```python
from build123d import *

# Parameters (mm, degrees)
SKETCH5_R           = 2.1
BOSS_EXTRUDE1_DEPTH = 125


with BuildPart() as part:
    # Sketch5 → Boss-Extrude1 (new body, symmetric)
    with BuildSketch(Plane(origin=(0, 0, 0), x_dir=(0, 0, -1), z_dir=(1, 0, 0))):
        with BuildLine():
            Line((-19.998019485, 4.9), (-18.198019485, 3.1))
            Line((-18.198019485, 3.1), (-18.198019485, 5.499339828))
            Line((-18.198019485, 5.499339828), (-16.558019485, 5.499339828))
            Line((-16.558019485, 5.499339828), (-13.9, 2.841320344))
            Line((-13.9, 2.841320344), (-13.9, -2.838679656))
            Line((-13.9, -2.838679656), (-16.558019485, -5.496699141))
            Line((-16.558019485, -5.496699141), (-18.198019485, -5.496699141))
            Line((-18.198019485, -5.496699141), (-18.198019485, -3.1))
            Line((-18.198019485, -3.1), (-19.998019485, -4.9))
            Line((-19.998019485, -4.9), (-19.998019485, -9))
            ThreePointArc((-19.998019485, -9), (-19.705126266, -9.707106781), (-18.998019485, -10))
            Line((-18.998019485, -10), (-14.9, -10))
            Line((-14.9, -10), (-13.1, -8.2))
            Line((-13.1, -8.2), (-15.5, -8.2))
            Line((-15.5, -8.2), (-15.5, -6.56))
            Line((-15.5, -6.56), (-12.84, -3.9))
            Line((-12.84, -3.9), (-7.16, -3.9))
            Line((-7.16, -3.9), (-4.5, -6.56))
            Line((-4.5, -6.56), (-4.5, -8.2))
            Line((-4.5, -8.2), (-6.9, -8.2))
            Line((-6.9, -8.2), (-5.1, -10))
            Line((-5.1, -10), (5.1, -10))
            Line((5.1, -10), (6.9, -8.2))
            Line((6.9, -8.2), (4.496038969, -8.2))
            Line((4.496038969, -8.2), (4.496038969, -6.56))
            Line((4.496038969, -6.56), (7.156038969, -3.9))
            Line((7.156038969, -3.9), (12.836038969, -3.9))
            Line((12.836038969, -3.9), (15.496038969, -6.56))
            Line((15.496038969, -6.56), (15.496038969, -8.2))
            Line((15.496038969, -8.2), (13.1, -8.2))
            Line((13.1, -8.2), (14.9, -10))
            Line((14.9, -10), (19.001980515, -10))
            ThreePointArc((19.001980515, -10), (19.709087297, -9.707106781), (20.001980515, -9))
            Line((20.001980515, -9), (20.001980515, -4.9))
            Line((20.001980515, -4.9), (18.201980515, -3.1))
            Line((18.201980515, -3.1), (18.201980515, -5.504621202))
            Line((18.201980515, -5.504621202), (16.561980515, -5.504621202))
            Line((16.561980515, -5.504621202), (13.9, -2.842640687))
            Line((13.9, -2.842640687), (13.9, 2.837359313))
            Line((13.9, 2.837359313), (16.561980515, 5.499339828))
            Line((16.561980515, 5.499339828), (18.201980515, 5.499339828))
            Line((18.201980515, 5.499339828), (18.201980515, 3.1))
            Line((18.201980515, 3.1), (20.001980515, 4.9))
            Line((20.001980515, 4.9), (20.001980515, 9))
            ThreePointArc((20.001980515, 9), (19.709087297, 9.707106781), (19.001980515, 10))
            Line((19.001980515, 10), (14.9, 10))
            Line((14.9, 10), (13.1, 8.2))
            Line((13.1, 8.2), (15.501320344, 8.2))
            Line((15.501320344, 8.2), (15.501320344, 6.56))
            Line((15.501320344, 6.56), (12.841320344, 3.9))
            Line((12.841320344, 3.9), (7.161320344, 3.9))
            Line((7.161320344, 3.9), (4.501320344, 6.56))
            Line((4.501320344, 6.56), (4.501320344, 8.2))
            Line((4.501320344, 8.2), (6.9, 8.2))
            Line((6.9, 8.2), (5.1, 10))
            Line((5.1, 10), (-5.1, 10))
            Line((-5.1, 10), (-6.9, 8.2))
            Line((-6.9, 8.2), (-4.501320344, 8.2))
            Line((-4.501320344, 8.2), (-4.501320344, 6.56))
            Line((-4.501320344, 6.56), (-7.161320344, 3.9))
            Line((-7.161320344, 3.9), (-12.841320344, 3.9))
            Line((-12.841320344, 3.9), (-15.501320344, 6.56))
            Line((-15.501320344, 6.56), (-15.501320344, 8.2))
            Line((-15.501320344, 8.2), (-13.1, 8.2))
            Line((-13.1, 8.2), (-14.9, 10))
            Line((-14.9, 10), (-18.998019485, 10))
            ThreePointArc((-18.998019485, 10), (-19.705126266, 9.707106781), (-19.998019485, 9))
            Line((-19.998019485, 9), (-19.998019485, 4.9))
        make_face()
        with Locations((-10, 0)):
            Circle(SKETCH5_R, mode=Mode.SUBTRACT)
        with Locations((10, 0)):
            Circle(SKETCH5_R, mode=Mode.SUBTRACT)
        Polygon((6.1, -2.84), (6.1, 2.84), (2.7, 6.24), (2.7, 8.2), (-2.7, 8.2), (-2.7, 6.24), (-6.1, 2.84), (-6.1, -2.84), (-2.7, -6.24), (-2.7, -8.2), (2.7, -8.2), (2.7, -6.24), align=None, mode=Mode.SUBTRACT)
        with BuildLine():
            Line((16.571320344, 8.2), (18.001980515, 8.2))
            ThreePointArc((18.001980515, 8.2), (18.143401872, 8.141421356), (18.201980515, 8))
            Line((18.201980515, 8), (18.201980515, 6.569339828))
            ThreePointArc((18.201980515, 6.569339828), (18.078517202, 6.384563922), (17.860559159, 6.427918472))
            Line((17.860559159, 6.427918472), (16.429898987, 7.858578644))
            ThreePointArc((16.429898987, 7.858578644), (16.386544437, 8.076536686), (16.571320344, 8.2))
        make_face(mode=Mode.SUBTRACT)
        with BuildLine():
            Line((16.571320344, -8.2), (18.001980515, -8.2))
            ThreePointArc((18.001980515, -8.2), (18.143401872, -8.141421356), (18.201980515, -8))
            Line((18.201980515, -8), (18.201980515, -6.569339828))
            ThreePointArc((18.201980515, -6.569339828), (18.078517202, -6.384563922), (17.860559159, -6.427918472))
            Line((17.860559159, -6.427918472), (16.429898987, -7.858578644))
            ThreePointArc((16.429898987, -7.858578644), (16.386544437, -8.076536686), (16.571320344, -8.2))
        make_face(mode=Mode.SUBTRACT)
        with BuildLine():
            Line((-17.860559159, 6.427918472), (-16.429898987, 7.858578644))
            ThreePointArc((-16.429898987, 7.858578644), (-16.386544437, 8.076536686), (-16.571320344, 8.2))
            Line((-16.571320344, 8.2), (-18.001980515, 8.2))
            ThreePointArc((-18.001980515, 8.2), (-18.143401872, 8.141421356), (-18.201980515, 8))
            Line((-18.201980515, 8), (-18.201980515, 6.569339828))
            ThreePointArc((-18.201980515, 6.569339828), (-18.078517202, 6.384563922), (-17.860559159, 6.427918472))
        make_face(mode=Mode.SUBTRACT)
        with BuildLine():
            Line((-16.571320344, -8.2), (-18.001980515, -8.2))
            ThreePointArc((-18.001980515, -8.2), (-18.143401872, -8.141421356), (-18.201980515, -8))
            Line((-18.201980515, -8), (-18.201980515, -6.569339828))
            ThreePointArc((-18.201980515, -6.569339828), (-18.078517202, -6.384563922), (-17.860559159, -6.427918472))
            Line((-17.860559159, -6.427918472), (-16.429898987, -7.858578644))
            ThreePointArc((-16.429898987, -7.858578644), (-16.386544437, -8.076536686), (-16.571320344, -8.2))
        make_face(mode=Mode.SUBTRACT)
    extrude(amount=BOSS_EXTRUDE1_DEPTH, both=True)


solid = part.part
```
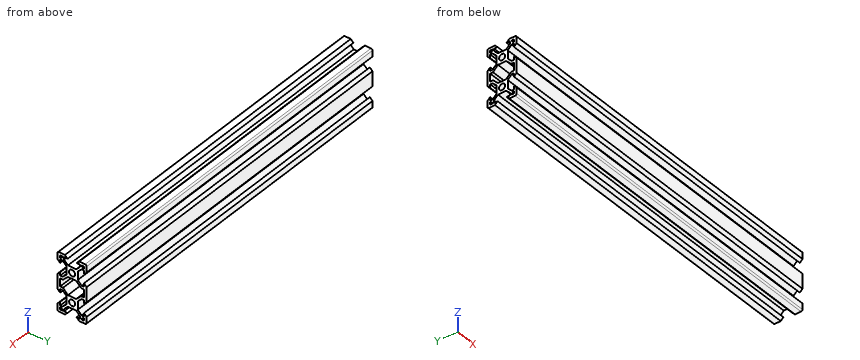
Geometry check sheet. Reference: the model listing, model coordinates, mm. Coordinates: 2 decimals unless noted, no trailing zeros. Order: outer loops, then holes, each group sorted by start corner. A loop starts at its lowest first (then second) coordinate and runs counter-clockwise, first axis right, second up. Notation, with made-up numbers: M -23.5,34 L 3.5,34 A16 ccw 3.5,60 Z; hole C -17.75,73.5 d5. An arc over 180 degrees is marked long. One line per question, with ' | ' between items. Start each with the question number.
Item 1: Material ranges on L1, parallel to Y at x = 16, z = -16; L2, parallel to Y at x = 55.5, z = -10; L3, parallel to Z at x = -43.5, y = -8.5, recorded low to high. Write a range as [from, to].
Item 2: Cross-section at A-A on y = 0. Enter the section's corners in (x, z), then the cut area to 3 significant figures.
Item 3: Gauge pin test, flat ends, axial feed: pin 1 (1.2 mm diameter, centred on x = -34.5, y = -4, fed in from +Z); pin 2 (2 mm diameter, centred on x = 70.5, z = -11, fed in from +Y); pin 3 (1 mm diameter, centred on x = 71.5, z = 11, fed in from -Y). Record the tip position at first contact, or that the pin passes through.
Item 4: Cross-section at C-C on x = -38.5. State how many separate pieces and enclosed holes the cut face has, then the cut area to 3 significant figures.
Item 5: Cross-section at B-B on z = 10. Enter the section's corners in (x, y), then the cut area to 3 significant figures.
Findings:
1) L1: y = [-10, -4.94], [4.94, 10] | L2: y = [-3.9, -2.1], [2.1, 3.9] | L3: z = [-20, -13.4], [-6.6, 6.6], [13.4, 20]
2) outline: M -125,-13.9 L 125,-13.9 L 125,-12.1 L -125,-12.1 Z; M -125,-7.9 L 125,-7.9 L 125,-6.1 L -125,-6.1 Z; M -125,6.1 L 125,6.1 L 125,7.9 L -125,7.9 Z; M -125,12.1 L 125,12.1 L 125,13.9 L -125,13.9 Z | area: 1,800 mm²
3) pin 1: stops at z = 19.7 | pin 2: stops at y = 3.9 | pin 3: stops at y = -3.9
4) separate pieces: 1 | enclosed holes: 7 | area: 285 mm²
5) outline: M -125,-3.9 L 125,-3.9 L 125,-2.1 L -125,-2.1 Z; M -125,2.1 L 125,2.1 L 125,3.9 L -125,3.9 Z | area: 900 mm²
